```python
from build123d import *

# Parameters (mm, degrees)
SKETCH1_R            = 43.456311094
BOSS_EXTRUDE10_DEPTH = 35
BOSS_EXTRUDE18_DEPTH = 7.421557236
SKETCH1_18_R         = 4.75
BOSS_EXTRUDE19_DEPTH = 2


with BuildPart() as part:
    # Sketch1 → Boss-Extrude10 (new body)
    with BuildSketch(Plane(origin=(0, 0, 0), x_dir=(1, 0, 0), z_dir=(0, 1, 0))):
        with Locations(Location((0, 0, 0), (0, 0, 270))):
            Circle(SKETCH1_R)
        with BuildLine():
            ThreePointArc((-10.807631289, 38.145414948), (0.461333582, 39.644227158), (11.692368711, 37.883586018))
            ThreePointArc((11.692368711, 37.883586018), (31.402087475, 24.203026213), (39.612178769, 1.659177136))
            Line((39.612178769, 1.659177136), (41.800929267, 1.659177136))
            Line((41.800929267, 1.659177136), (41.800929267, -1.659177136))
            Line((41.800929267, -1.659177136), (39.612178769, -1.659177136))
            ThreePointArc((39.612178769, -1.659177136), (0, -39.6469113), (-39.612178769, -1.659177136))
            Line((-39.612178769, -1.659177136), (-41.800929267, -1.659177136))
            Line((-41.800929267, -1.659177136), (-41.800929267, 1.659177136))
            Line((-41.800929267, 1.659177136), (-39.612178769, 1.659177136))
            ThreePointArc((-39.612178769, 1.659177136), (-31.118333808, 24.566784011), (-10.807631289, 38.145414948))
        make_face(mode=Mode.SUBTRACT)
    extrude(amount=BOSS_EXTRUDE10_DEPTH)

    # Sketch1_17 → Boss-Extrude18 (add)
    with BuildSketch(Plane(origin=(0, 0, 0), x_dir=(1, 0, 0), z_dir=(0, 1, 0))):
        with BuildLine():
            Line((41.800929267, 1.659177136), (39.612178769, 1.659177136))
            ThreePointArc((39.612178769, 1.659177136), (39.638227216, 0.829770317), (39.6469113, 0))
            ThreePointArc((39.6469113, 0), (39.638227216, -0.829770317), (39.612178769, -1.659177136))
            Line((39.612178769, -1.659177136), (41.800929267, -1.659177136))
            Line((41.800929267, -1.659177136), (41.800929267, 1.659177136))
        make_face()
        with BuildLine():
            ThreePointArc((-39.612178769, -1.659177136), (-39.6469113, 0), (-39.612178769, 1.659177136))
            Line((-39.612178769, 1.659177136), (-41.800929267, 1.659177136))
            Line((-41.800929267, 1.659177136), (-41.800929267, -1.659177136))
            Line((-41.800929267, -1.659177136), (-39.612178769, -1.659177136))
        make_face()
    extrude(amount=BOSS_EXTRUDE18_DEPTH)

    # Sketch1_18 → Boss-Extrude19 (add)
    with BuildSketch(Plane(origin=(0, 0, 0), x_dir=(1, 0, 0), z_dir=(0, 1, 0))):
        with BuildLine():
            Line((11.692368711, 37.883586018), (11.692368711, 32.635924628))
            ThreePointArc((11.692368711, 32.635924628), (11.399475492, 31.928817847), (10.692368711, 31.635924628))
            Line((10.692368711, 31.635924628), (-9.807631289, 31.635924628))
            ThreePointArc((-9.807631289, 31.635924628), (-10.51473807, 31.928817847), (-10.807631289, 32.635924628))
            Line((-10.807631289, 32.635924628), (-10.807631289, 38.145414948))
            ThreePointArc((-10.807631289, 38.145414948), (-0.461333582, -39.644227158), (11.692368711, 37.883586018))
        make_face()
        with Locations(Location((0, 0, 0), (0, 0, 270))):
            Circle(SKETCH1_18_R, mode=Mode.SUBTRACT)
    extrude(amount=BOSS_EXTRUDE19_DEPTH)


solid = part.part
```
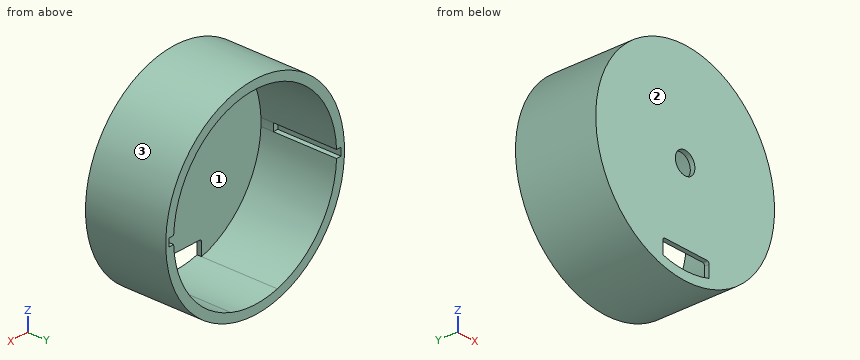
CAD build for the part. Positions are in the model's coordinates, mm. Face numbers are marked on the shaded views. Coordinates: 2 decimals unless noted, no trailing zeros. Order: outer loops, then holes, each group sorted by start corner. A loop starts at its lowest first (then second) coordinate and runs counter-clockwise, first axis right, second up.
(1) Saw through at C-C, the plane z = -17.5. Write the cut outline in (x, y), and give its area (3 significant figures).
Solution:
outline: (-39.78, 0) - (39.78, 0) - (39.78, 35) - (35.58, 35) - (35.58, 2) - (-35.58, 2) - (-35.58, 35) - (-39.78, 35) - close
area: 436 mm2
(2) Pin check, flat tips, straight feed: pin 1 Ø2 at (x, z) = (5, -11.5) entering from +Y; pin 2 Ø4 at (x, y) = (-12.5, 6.5) entering from -Z; pin 3 Ø2.5 at (x, z) = (-40, 0) entering from +Y. Stop position of each tip, or through.
Solution:
pin 1: stops at y = 2
pin 2: stops at z = -42.17
pin 3: stops at y = 7.42
(3) Drill centre lines: L1, parallel to X at y = 1.15, z = 0; L2, parallel to X at y = 19.5, z = 0.5; L3, parallel to Y at x = 19, z = -1.5. Where is each one in solid material? Low to high.
Solution:
L1: x = -43.46 to -4.75, 4.75 to 43.46
L2: x = -43.45 to -41.8, 41.8 to 43.45
L3: y = 0 to 2
(4) Mould opens along X. For the marked faces 1, 2 and 3 say: released by +X, released by -X, zero draft, split by the parting line, or undercut.
Solution:
face 1: undercut
face 2: zero draft
face 3: split by the parting line
(5) Saw through at A-A, the plane x = 0. Write the cut outline in (y, z).
Solution:
outline: (0, -43.46) - (35, -43.46) - (35, -39.65) - (0, -39.65) - close; (0, -31.64) - (2, -31.64) - (2, -4.75) - (0, -4.75) - close; (0, 4.75) - (2, 4.75) - (2, 39.65) - (35, 39.65) - (35, 43.46) - (0, 43.46) - close
(6) Saw through at D-D, the plane x = -15. Write the cut outline in (y, z), and give its area (3 significant figures).
Solution:
outline: (0, -40.79) - (35, -40.79) - (35, -36.7) - (2, -36.7) - (2, 36.7) - (35, 36.7) - (35, 40.79) - (0, 40.79) - close
area: 433 mm2
(7) Saw through at B-B, the plane y = 6. Write the cut outline in (x, z), and give its area (3 significant figures).
Solution:
outline: circle Ø86.91 at (0, 0); hole circle Ø79.29 at (0, 0)
area: 995 mm2
